from build123d import *

# Parameters (mm, degrees)
F0_R     = 21
F1_DEPTH = 5.5
F2_DEPTH = 3


# Not quite as in the source:
# - a feature of the source that left no trace in its solid (it failed there, or was rolled back) is left out


with BuildPart() as f1:
    # F0 (on Top) → F1 (new body)
    with BuildSketch(Plane.XY):
        with BuildLine():
            ThreePointArc((25.8795285892, -2.5), (25.9698646831, -1.2514504945), (26, 0))
            ThreePointArc((26, 0), (25.9698646831, 1.2514504945), (25.8795285892, 2.5))
            ThreePointArc((25.8795285892, 2.5), (-26, 0), (25.8795285892, -2.5))
        make_face()
        Circle(F0_R, mode=Mode.SUBTRACT)
        with BuildLine():
            ThreePointArc((25.8795285892, 2.5), (25.9698646831, 1.2514504945), (26, 0))
            ThreePointArc((26, 0), (25.9698646831, -1.2514504945), (25.8795285892, -2.5))
            Line((25.8795285892, -2.5), (48, -2.5))
            Line((48, -2.5), (48, 0))
            Line((48, 0), (48, 2.5))
            Line((48, 2.5), (25.8795285892, 2.5))
        make_face()
        Circle(F0_R)
    extrude(amount=F1_DEPTH)

    # F0 (on Top) → F2 (cut)
    with BuildSketch(Plane.XY):
        Circle(F0_R)
    extrude(amount=F2_DEPTH, mode=Mode.SUBTRACT)


solid = f1.part
Can you work these out from the model? Positions are in its coordinate system, mm. A direction names the side the tool comes from. Coordinates: 2 decimals unless noted, no trailing zeros. Order: outer loops, then holes, each group sorted by start corner. A loop starts at its lowest first (then second) coordinate and runs counter-clockwise, first axis right, second up. Notation, with made-up numbers: (22.25, -19.75) -> (57.25, -19.75) arc R22 ccw to (57.25, 3.25) -> close; hole circle Ø8 at (-19.5, 65). An arc over 180 degrees is marked (long way). Use one line per item in the form item = value.
Q1. We'd pull the mould along Y, two halves only. Please class faces 1 (the face through (0, 0, 3)), 2 (the face through (2, 0, 5.5)), 3 (the face through (37, -2.5, 3)): released by +Y, released by -Y, zero draft, split by the parting line, or undercut.
From the geometry:
face_1 = undercut
face_2 = zero draft
face_3 = released by -Y
Q2. I need wall thicknesses on L1, parallel to Y at x = 0, z = 1.15; L2, parallel to Y at x = 26, z = 1.6; L3, parallel to Z at x = 2, y = -20. Which ranges of each line are inside material? Lowest first, please.
From the geometry:
L1 = -26 to -21, 21 to 26
L2 = -2.5 to 2.5
L3 = 3 to 5.5
Q3. Imagine slicing it at A-A, the plane z = 1.6. List the corners of the cut face in (x, y) for me, then the cut area to 3 significant figures.
From the geometry:
outline = (25.88, -2.5) -> (48, -2.5) -> (48, 2.5) -> (25.88, 2.5) arc R26 ccw (long way) to start; hole circle Ø42 at (0, 0)
area = 848 mm²
Q4. Which directions (+Z, -Z, +X, -X, +Y, -Y) give clear straight access to the entire face, cutting with the end or side of a thin tool? Please do faces 4 (the face through (20.03, 6.31, 1.48)), 5 (the face through (37, 2.5, 3)), 6 (the face through (48, 0, 3)).
From the geometry:
face_4 = -Z
face_5 = +Z, -Z, +X, +Y
face_6 = +Z, -Z, +X, +Y, -Y
Q5. Imagine slicing it at C-C, the plane x = 0. List the corners of the cut face in (y, z) for me, then the cut area to 3 significant figures.
From the geometry:
outline = (-26, 0) -> (-21, 0) -> (-21, 3) -> (21, 3) -> (21, 0) -> (26, 0) -> (26, 5.5) -> (-26, 5.5) -> close
area = 160 mm²
Q6. Will these pins go through, and if not, where does the flat tip stop? P1, Ø2, axis at y = 10.5, z = 1.5, coming from the -X side; P2, Ø21, axis at x = 4.5, y = -8, coming from the -Z side; P3, Ø3, axis at y = 20.5, z = 1, coming from the -X side.
From the geometry:
P1 = -24.2
P2 = 3
P3 = -17.75
Q7. Imagine slicing it at B-B, the plane y = 0. List the corners of the cut face in (x, z) for me.
From the geometry:
outline = (-26, 0) -> (-21, 0) -> (-21, 3) -> (21, 3) -> (21, 0) -> (48, 0) -> (48, 5.5) -> (-26, 5.5) -> close
Q8. Imagine slicing it at D-D, the plane x = 29.5. List the corners of the cut face in (y, z) for me.
From the geometry:
outline = (-2.5, 0) -> (2.5, 0) -> (2.5, 5.5) -> (-2.5, 5.5) -> close
